Could you check a few things on this model? Use its own coordinates, in mm. Face numbers are marked on the shaded views. A direction names the side the tool comes from. Coordinates: 2 decimals unless noted, no trailing zeros. Order: outer loops, then holes, each group sorted by start corner. A loop starts at its lowest first (then second) coordinate and runs counter-clockwise, first axis right, second up. Notation, with made-up numbers: (70.25, 30.5) -> (97.25, 30.5) arc R16 ccw to (97.25, 42.5) -> close; hole circle Ø2 at (-11, 13.25). An arc over 180 degrees is marked (long way). Put each result on its own line as item: value. Start each with the question number.
Q1. If we section it at B-B (z = -19.25): Please give me the cut outline in (x, y).
Q2. Please list where these lines run through material, in increasing order: line 1 along X through (y, z) = (-1, -23); line 2 along X through (y, z) = (10.75, -8.5); line 3 along Z through (x, y) = (-5.75, 21.5).
Q3. If we section it at D-D (y = 7): Please give me the cut outline in (x, z), and give its area (3 significant figures).
Q4. For the marked faces 4, 5, 6, 7 and 8, which set-ups out of +Z, -Z, +X, -X, +Y, -Y let a thin tool reach every point of the face, with its end or its side?
Q5. We'd pull the mould along X, two halves only. Please class the marked faces 1, 2 and 3: +X half, -X half, draft (parallel to the pull), parting line (faces both ways), or undercut.
Q6. If we section it at A-A (z = -7.1): Count the separate pieces of the cut face and the enclosed holes in it, and give its area (3 significant figures).
Q7. If we section it at C-C (x = -13.5): Please give me the cut outline in (y, z).
Q8. Will these pins go through, and if not, where does the flat tip stop? pin 1 (1.8 mm diameter, centred on y = 20, z = -8.5, fed in from -X); pin 2 (0.9 mm diameter, centred on x = -12, y = -1.5, fed in from +Z); pin 3 (2.5 mm diameter, centred on y = 15, z = -7.1, fed in from +X); pin 4 (0.8 mm diameter, centred on x = 8, y = 21, fed in from -Z).
from build123d import *

# Parameters (mm, degrees)
EXTRUDE_1_DEPTH           = 25
SKETCH_2_W                = 19
SKETCH_2_H                = 28
SKETCH_2_R                = 1.5
EXTRUDE_2_DEPTH           = 3
SKETCH_3_W                = 1
SKETCH_3_H                = 6
CUT_EXTRUDE_1_DEPTH       = 15
SKETCH_4_R                = 0.9
CUT_EXTRUDE_2_DEPTH       = 19
FILLET_1_R                = 3
EXTRUDE_3_DEPTH           = 2
EXTRUDE_4_DEPTH           = 5
FILLET_2_R                = 3
CHAMFER_1_SIZE            = 0.5
EXTRUDE_5_DEPTH           = 3
HOLE_WIZARD_3_0_3_1_D     = 3
HOLE_WIZARD_3_0_3_1_DEPTH = 3


with BuildPart() as part:
    # 草图1 → 凸台-拉伸1 (new body)
    with BuildSketch(Plane(origin=(0, 0, 0), x_dir=(1, 0, 0), z_dir=(0, 1, 0))):
        Polygon((-9.5, 10.1), (-9.5, 0), (9.5, 0), (9.5, 10.1), (5, 10.1), (5, 8.1), (6.5, 8.1), (6.5, 2), (-6.5, 2), (-6.5, 8.1), (-5, 8.1), (-5, 10.1), align=None)
    extrude(amount=EXTRUDE_1_DEPTH)

    # 草图2 → 凸台-拉伸2 (add)
    with BuildSketch(Plane.XZ):
        with Locations((0, -14)):
            Rectangle(SKETCH_2_W, SKETCH_2_H)
        with Locations((4, -25)):
            Circle(SKETCH_2_R, mode=Mode.SUBTRACT)
        with Locations((-4, -25)):
            Circle(SKETCH_2_R, mode=Mode.SUBTRACT)
    extrude(amount=EXTRUDE_2_DEPTH)

    # 草图3 → 切除-拉伸1 (cut)
    with BuildSketch(Plane(origin=(0, 25, 0), x_dir=(1, 0, 0), z_dir=(0, 1, 0))):
        with Locations((-8, 7.1)):
            Rectangle(SKETCH_3_W, SKETCH_3_H)
        with Locations((8, 7.1)):
            Rectangle(SKETCH_3_W, SKETCH_3_H)
    extrude(amount=-CUT_EXTRUDE_1_DEPTH, mode=Mode.SUBTRACT)

    # 草图4 → 切除-拉伸2 (cut)
    with BuildSketch(Plane.ZY.offset(9.5)):
        with Locations((-7.1, 15)):
            Circle(SKETCH_4_R)
    extrude(amount=-CUT_EXTRUDE_2_DEPTH, mode=Mode.SUBTRACT)

    # 圆角1
    fillet_1_edges = [part.edges().sort_by_distance(p)[0] for p in [
        (9.5, -1.5, -28),
        (-9.5, -1.5, -28),
    ]]
    fillet(fillet_1_edges, radius=FILLET_1_R)

    # 草图5 → 凸台-拉伸3 (add)
    with BuildSketch(Plane.ZY.offset(9.5)):
        Polygon((-10.1, 0), (-10.1, 6), (-20.1, 0), align=None)
    extrude_3 = extrude(amount=-EXTRUDE_3_DEPTH)

    # 镜向1: 凸台-拉伸3 across plane
    add(extrude_3.mirror(Plane(origin=(0, 0, 0), x_dir=(0, 0, 1), z_dir=(1, 0, 0))))

    # 草图6 → 凸台-拉伸4 (add)
    with BuildSketch(Plane(origin=(0, 0, 0), x_dir=(1, 0, 0), z_dir=(0, 1, 0))):
        Polygon((-6.5, 2), (6.5, 2), (6.5, 8.1), (5, 8.1), (5, 10.1), (-5, 10.1), (-5, 8.1), (-6.5, 8.1), align=None)
    extrude(amount=EXTRUDE_4_DEPTH)

    # 圆角2
    fillet_2_edges = [part.edges().sort_by_distance(p)[0] for p in [
        (0, -3, 0),
    ]]
    fillet(fillet_2_edges, radius=FILLET_2_R)

    # 倒角1
    chamfer_1_edges = [part.edges().sort_by_distance(p)[0] for p in [
        (5, 25, -9.1),
        (5.75, 25, -8.1),
        (6.5, 25, -5.05),
        (0, 25, -2),
        (-6.5, 25, -5.05),
        (-5.75, 25, -8.1),
        (-5, 25, -9.1),
    ]]
    chamfer(chamfer_1_edges, length=CHAMFER_1_SIZE)

    # 草图7 → 凸台-拉伸5 (add)
    with BuildSketch(Plane(origin=(0, 0, 0), x_dir=(1, 0, 0), z_dir=(0, 1, 0))):
        with BuildLine():
            Line((6.5, 28), (-15.797958971, 28))
            ThreePointArc((-15.797958971, 28), (-17.919279315, 27.121320344), (-18.797958971, 25))
            Line((-18.797958971, 25), (-18.797958971, 23.1))
            ThreePointArc((-18.797958971, 23.1), (-17.919279315, 20.978679656), (-15.797958971, 20.1))
            Line((-15.797958971, 20.1), (6.5, 20.1))
            Line((6.5, 20.1), (6.5, 28))
        make_face()
    extrude(amount=-EXTRUDE_5_DEPTH)

    # Ø3.0 (3) 直径孔1
    with Locations(Plane(origin=(0, 0, 0), x_dir=(1, 0, 0), z_dir=(0, 1, 0))):
        with Locations((-5.797958971, 23), (-13.797958971, 23)):
            Hole(HOLE_WIZARD_3_0_3_1_D / 2, depth=HOLE_WIZARD_3_0_3_1_DEPTH)


solid = part.part
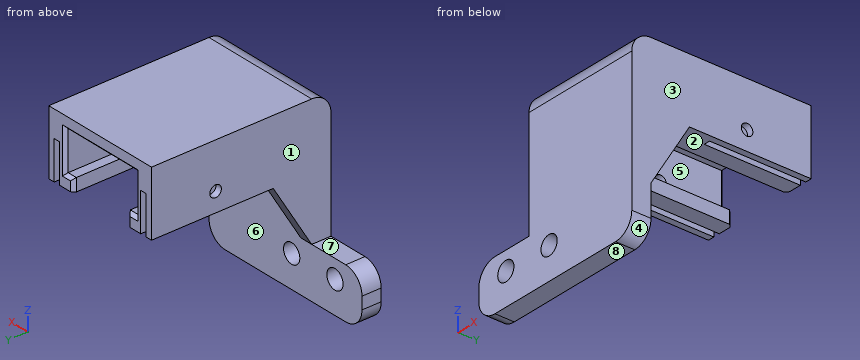
The answers:
1. outline: (-9.5, -3) -> (9.5, -3) -> (9.5, 0.51) -> (7.5, 0.51) -> (7.5, 0) -> (-7.5, 0) -> (-7.5, 0.51) -> (-9.5, 0.51) -> close
2. line 1: -18.8 to -15.3, -12.3 to -7.3, -4.3 to 9.5
2. line 2: -9.5 to -8.5, -7.5 to -5, 5 to 7.5, 8.5 to 9.5
2. line 3: -10.1 to -8.1, -2 to 0
3. outline: (-9.5, -10.1) -> (-5, -10.1) -> (-5, -8.1) -> (-6.5, -8.1) -> (-6.5, -2) -> (6.5, -2) -> (6.5, -8.1) -> (5, -8.1) -> (5, -10.1) -> (9.5, -10.1) -> (9.5, 0) -> (-9.5, 0) -> close
3. area: 92.6 mm^2
4. face 4: -Z, +X, +Y, -Y
4. face 5: +Y
4. face 6: -Z, +Y
4. face 7: +Z, -X, +Y, -Y
4. face 8: -Z, +X, -X, +Y, -Y
5. face 1: -X half
5. face 2: undercut
5. face 3: +X half
6. separate pieces: 5
6. enclosed holes: 0
6. area: 235 mm^2
7. outline: (-3, -28) -> (0, -28) -> (0, -24.47) -> (-3, -24.47) -> close; (-3, -21.53) -> (0, -21.53) -> (0, -20.1) -> (-3, -20.1) -> close
8. pin 1: x = -9.5
8. pin 2: z = -20.1
8. pin 3: x = 9.5
8. pin 4: z = -4.1
